```python
from build123d import *

# Parameters (mm, degrees)
SKETCH1_R                 = 8.25
BOSS_EXTRUDE1_DEPTH       = 9
M4X0_7_TAPPED_HOLE1_D     = 3.3
M4X0_7_TAPPED_HOLE1_DEPTH = 11
M4X0_7_TAPPED_HOLE1_TIP   = 0.991420021
CUT_EXTRUDE4_DEPTH        = 15


with BuildPart() as part:
    # Sketch1 → Boss-Extrude1 (new body)
    with BuildSketch(Plane(origin=(0, 0, 0), x_dir=(1, 0, 0), z_dir=(0, 1, 0))):
        with BuildLine():
            Line((39.406576406, 4.5), (39.406576406, -4.5))
            Line((39.406576406, -4.5), (34.406576406, -4.5))
            ThreePointArc((34.406576406, -4.5), (21.47943012, -6.646481156), (9.939677628, -12.855555556))
            ThreePointArc((9.939677628, -12.855555556), (-16.25, 0), (9.939677628, 12.855555556))
            ThreePointArc((9.939677628, 12.855555556), (21.47943012, 6.646481156), (34.406576406, 4.5))
            Line((34.406576406, 4.5), (39.406576406, 4.5))
        make_face()
        with Locations(Location((0, 0, 0), (0, 0, 270))):
            Circle(SKETCH1_R, mode=Mode.SUBTRACT)
    extrude(amount=BOSS_EXTRUDE1_DEPTH)

    # M4x0.7 Tapped Hole1
    with Locations(Plane(origin=(39.406576406, 0, 0), x_dir=(0, 0, -1), z_dir=(1, 0, 0))):
        with Locations((0, 4.5)):
            Hole(M4X0_7_TAPPED_HOLE1_D / 2, depth=M4X0_7_TAPPED_HOLE1_DEPTH)
            with Locations((0, 0, -(M4X0_7_TAPPED_HOLE1_DEPTH + M4X0_7_TAPPED_HOLE1_TIP / 2))):  # 118° drill point
                Cone(0, M4X0_7_TAPPED_HOLE1_D / 2, M4X0_7_TAPPED_HOLE1_TIP, mode=Mode.SUBTRACT)

    # Sketch11 → Cut-Extrude4 (cut)
    with BuildSketch(Plane(origin=(39.406576406, 0, 0), x_dir=(0, 0, -1), z_dir=(1, 0, 0))):
        Polygon((-1.5, 9), (0, 10.5), (-6, 10.5), (-6, 4.5), (-4.5, 6), (-4.5, 9), align=None)
        Polygon((-4.5, 6), (-1.5, 9), (-4.5, 9), align=None)
        Polygon((6, 10.5), (0, 10.5), (1.5, 9), (4.5, 9), (4.5, 6), (6, 4.5), align=None)
        Polygon((4.5, 9), (1.5, 9), (4.5, 6), align=None)
        Polygon((4.5, 0), (4.5, 3), (1.5, 0), align=None)
        Polygon((6, -1.5), (6, 4.5), (4.5, 3), (4.5, 0), (1.5, 0), (0, -1.5), align=None)
        Polygon((-1.5, 0), (-4.5, 3), (-4.5, 0), align=None)
        Polygon((-4.5, 3), (-6, 4.5), (-6, -1.5), (0, -1.5), (-1.5, 0), (-4.5, 0), align=None)
    extrude(amount=-CUT_EXTRUDE4_DEPTH, mode=Mode.SUBTRACT)


solid = part.part
```
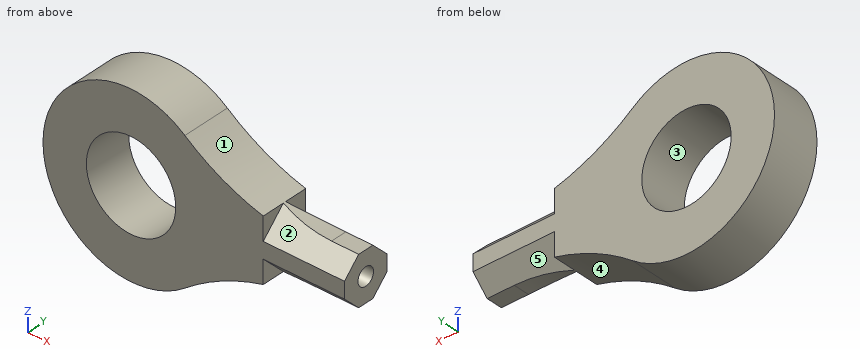
The listing builds one solid part. Answer for the finished solid, in the listing's coordinates (mm). Face numbers are marked on the shaded views. A direction names the side the tool comes from. Round coordinates to 2 decimals unless told otherwise and drop trailing zeros. Order: outer loops, then holes, each group sorted by start corner. A loop starts at its lowest first (then second) coordinate and runs counter-clockwise, first axis right, second up. Notation, with made-up numbers: (-7, 80) - (5, 80) arc R26 ccw to (5, 119) - close; hole circle Ø10 at (16, -4). An arc over 180 degrees is marked (long way). Put each result on its own line as item: value. Start each with the question number.
(1) Find section C-C (z = 6.5). Give the vertices of the cut face in (x, y), plus the area to 3 significant figures.
(2) Determine the mould class of the marked faces 3, 4 and 5 for opening direction X: released by +X, released by -X, zero draft, split by the parting line, or undercut.
(3) Find section D-D (x = 33). Give the vertices of the cut face in (y, z).
(4) Straight lines are drawn through the part: probe 1 along X at (y, z) = (2.75, 0); probe 2 along Y at (x, z) = (33, 0); probe 3 along Z at (x, y) = (33.75, 4.5). For each, find the intervals that lie inside material, in ascending order. Write a range as from..to.
(5) Given P1, Ø5, axis at y = 6.5, z = -10.5, coming from the -X side; P2, Ø5, axis at y = 8, z = 11, coming from the -X side; P3, Ø3, axis at y = 4.5, z = 0, coming from the +X side, each flat-ended and moving along its own axis, determine where each tip first touches the part or whether it passes through.
(6) For the marked faces 1 and 2, determine the directions among +Z, -Z, +X, -X, +Y, -Y from which every point of the face is accessible in a straight line to the end or side of a thin tool.
(7) Find section A-A (x = 0). Give the vertices of the cut face in (y, z), plus the area to 3 significant figures.
(8) Find section B-B (y = 6.75). Give the vertices of the cut face in (x, z), plus the area to 3 significant figures.
Reply:
1. outline: (-14.89, 0) - (-5.08, 0) - (-5.08, 9) - (-14.89, 9) - close; (5.08, 0) - (21.92, 0) - (21.92, 9) - (5.08, 9) - close
1. area: 240 mm^2
2. face 3: undercut
2. face 4: released by +X
2. face 5: zero draft
3. outline: (0, -1.5) - (3.02, -4.52) - (5.98, -4.52) - (9, -1.5) - (9, 1.5) - (5.98, 4.52) - (3.02, 4.52) - (0, 1.5) - close; hole circle Ø3.3 at (4.5, 0)
4. probe 1: -16.25..-8.25, 8.25..39.41
4. probe 2: 0..2.85, 6.15..9
4. probe 3: -4.51..-1.65, 1.65..4.51
5. P1: x = -14.14
5. P2: x = -13.85
5. P3: x = 28.32
6. face 1: +Z, +X, +Y, -Y
6. face 2: +Z, +X, -Y
7. outline: (0, -16.25) - (9, -16.25) - (9, -8.25) - (0, -8.25) - close; (0, 8.25) - (9, 8.25) - (9, 16.25) - (0, 16.25) - close
7. area: 144 mm^2
8. outline: (9.94, -12.86) arc R40 cw to (24.41, -5.77) - (24.41, -3.75) - (39.41, -3.75) - (39.41, 3.75) - (24.41, 3.75) - (24.41, 5.77) arc R40 cw to (9.94, 12.86) arc R16.25 ccw (long way) to start; hole circle Ø16.5 at (0, 0)
8. area: 867 mm^2
